```python
from build123d import *

# Parameters (mm, degrees)
SKETCH1_W               = 47
SKETCH1_H               = 26.5
SKETCH1_W_2             = 41
SKETCH1_H_2             = 20.5
BOSS_EXTRUDE1_DEPTH     = 31
CUT_EXTRUDE2_DEPTH      = 31
SKETCH4_W               = 34.29807853
SKETCH4_H               = 20
BOSS_EXTRUDE2_DEPTH     = 10
SKETCH5_W               = 5
SKETCH5_H               = 17.5
CUT_EXTRUDE3_DEPTH      = 45
CUT_EXTRUDE4_DEPTH      = 64
CUT_EXTRUDE4_DEPTH_BACK = 45
SKETCH6_R               = 4.31945574
SKETCH7_W               = 8.63891148
SKETCH7_H               = 8.75
CUT_EXTRUDE5_DEPTH      = 10
FILLET2_START           = -23.25
FILLET2_DEPTH           = 5
SKETCH8_W               = 26.5
SKETCH8_H               = 5.5
CUT_EXTRUDE6_DEPTH      = 55
BOSS_EXTRUDE3_DEPTH     = 2.4
SKETCH10_W              = 5
SKETCH10_H              = 20
CUT_EXTRUDE7_DEPTH      = 39.4
FILLET4_R               = 5


with BuildPart() as part:
    # Sketch1 → Boss-Extrude1 (new body)
    with BuildSketch(Plane(origin=(0, 0, 0), x_dir=(1, 0, 0), z_dir=(0, 1, 0))):
        Rectangle(SKETCH1_W, SKETCH1_H)
        Rectangle(SKETCH1_W_2, SKETCH1_H_2, mode=Mode.SUBTRACT)
    extrude(amount=BOSS_EXTRUDE1_DEPTH)

    # Sketch3 → Cut-Extrude2 (cut)
    with BuildSketch(Plane(origin=(0, 31, 0), x_dir=(1, 0, 0), z_dir=(0, 1, 0))):
        Polygon((-19.366144394, -10.25), (-20.5, -13.25), (0, -13.25), (0, -10.25), align=None)
        Polygon((0, -10.25), (0, -13.25), (20.5, -13.25), (19.366144394, -10.25), align=None)
    extrude(amount=-CUT_EXTRUDE2_DEPTH, mode=Mode.SUBTRACT)

    # Sketch4 → Boss-Extrude2 (add)
    with BuildSketch(Plane(origin=(0, 0, -13.25), x_dir=(-1, 0, 0), z_dir=(0, 0, -1))):
        with Locations((0, 15.5)):
            Rectangle(SKETCH4_W, SKETCH4_H)
    extrude(amount=BOSS_EXTRUDE2_DEPTH)

    # Sketch5 → Cut-Extrude3 (cut)
    with BuildSketch(Plane(origin=(17.149039265, 0, 0), x_dir=(0, 0, -1), z_dir=(1, 0, 0))):
        with Locations((15.75, 14.25)):
            Rectangle(SKETCH5_W, SKETCH5_H)
    extrude(amount=-CUT_EXTRUDE3_DEPTH, mode=Mode.SUBTRACT)

    # Sketch6 → Cut-Extrude4 (cut, two sides: drawn at the far end of the back side and taken through both)
    with BuildSketch(Plane.XY.offset(-18.25).offset(-CUT_EXTRUDE4_DEPTH_BACK)):
        with Locations(Location((0, 14.25, 0), (0, 0, 180))):
            Circle(SKETCH6_R)
    extrude(amount=CUT_EXTRUDE4_DEPTH + CUT_EXTRUDE4_DEPTH_BACK, mode=Mode.SUBTRACT)

    # Sketch7 → Cut-Extrude5 (cut)
    with BuildSketch(Plane(origin=(0, 0, -23.25), x_dir=(-1, 0, 0), z_dir=(0, 0, -1))):
        with Locations((0, 9.875)):
            Rectangle(SKETCH7_W, SKETCH7_H)
    extrude(amount=-CUT_EXTRUDE5_DEPTH, mode=Mode.SUBTRACT)

    # Fillet2: read off the stored shape, not the designer's step
    # Fillet2 outline → Fillet2 (cut)
    with BuildSketch(Plane.XY.offset(FILLET2_START)):
        with BuildLine():
            ThreePointArc((-4.31945574, 14.25), (-4.315331507, 14.438711079), (-4.302966685, 14.627061794))
            ThreePointArc((-4.302966685, 14.627061794), (-7.509401663, 8.126758445), (-14.264792768, 5.5))
            Line((-14.264792768, 5.5), (-4.31945574, 5.5))
            Line((-4.31945574, 5.5), (-4.31945574, 14.25))
        make_face()
        with BuildLine():
            ThreePointArc((14.264792768, 5.5), (7.509401663, 8.126758445), (4.302966685, 14.627061794))
            ThreePointArc((4.302966685, 14.627061794), (4.315331507, 14.438711079), (4.31945574, 14.25))
            Line((4.31945574, 14.25), (4.31945574, 5.5))
            Line((4.31945574, 5.5), (14.264792768, 5.5))
        make_face()
    extrude(amount=FILLET2_DEPTH, mode=Mode.SUBTRACT)

    # Sketch8 → Cut-Extrude6 (cut)
    with BuildSketch(Plane(origin=(23.5, 0, 0), x_dir=(0, 0, -1), z_dir=(1, 0, 0))):
        with Locations((0, 2.75)):
            Rectangle(SKETCH8_W, SKETCH8_H)
    extrude(amount=-CUT_EXTRUDE6_DEPTH, mode=Mode.SUBTRACT)

    # Sketch9 → Boss-Extrude3 (add)
    with BuildSketch(Plane.XY.offset(-18.25)):
        with BuildLine():
            Line((-17.149039265, 23), (17.149039265, 23))
            Line((17.149039265, 23), (17.149039265, 5.5))
            Line((17.149039265, 5.5), (14.264792768, 5.5))
            ThreePointArc((14.264792768, 5.5), (7.509401663, 8.126758445), (4.302966685, 14.627061794))
            ThreePointArc((4.302966685, 14.627061794), (0, 18.56945574), (-4.302966685, 14.627061794))
            ThreePointArc((-4.302966685, 14.627061794), (-7.509401663, 8.126758445), (-14.264792768, 5.5))
            Line((-14.264792768, 5.5), (-17.149039265, 5.5))
            Line((-17.149039265, 5.5), (-17.149039265, 23))
        make_face()
    extrude(amount=BOSS_EXTRUDE3_DEPTH)

    # Sketch10 → Cut-Extrude7 (cut)
    with BuildSketch(Plane(origin=(17.149039265, 0, 0), x_dir=(0, 0, -1), z_dir=(1, 0, 0))):
        with Locations((20.75, 15.5)):
            Rectangle(SKETCH10_W, SKETCH10_H)
    extrude(amount=-CUT_EXTRUDE7_DEPTH, mode=Mode.SUBTRACT)

    # Fillet4
    fillet4_edges = [part.edges().sort_by_distance(p)[0] for p in [
        (0, 25.5, -13.25),
    ]]
    fillet(fillet4_edges, radius=FILLET4_R - 0.0001)  # a hair under: the kernel refuses the full size


solid = part.part
```
Can you work these out from the model? Positions are in its coordinate system, mm. A direction names the side the tool comes from. Round coordinates to 2 decimals unless told otherwise and drop trailing zeros. Loops run counter-clockwise (first coordinate to the right, second up) from the corner with the lowest first, then second, coordinate; pieces in that order, holes last.
Item 1: Suppose I cut it at D-D, the plane y = 8. Write out the boundary of the cut face in (x, z), then the cut area to 3 significant figures.
Item 2: Please list where these lines run through material, in increasing order: L1, parallel to X at y = 16, z = -6.5; L2, parallel to Z at x = 13, y = 13.25; L3, parallel to Y at x = 0, z = -12.
Item 3: Which directions (+Z, -Z, +X, -X, +Y, -Y) give clear straight access to the entire face, cutting with the end or side of a thin tool? Please do faces 1 (the flat face through (-20.5, 18, 0)), 2 (the flat face through (17.149, 18, -16)), 3 (the cylindrical face through (7.586, 8.057, -17.067)), 4 (the flat face through (0, 23, -15)).
Item 4: Will these pins go through, and if not, where does the flat tip stop? pin 1 Ø4 at (x, y) = (8.5, 28) entering from +Z; pin 2 Ø0.8 at (x, z) = (-4, -15) entering from -Y.
Item 5: Suppose I cut it at B-B, the plane y = 17.5. Write out the boundary of the cut face in (x, z).
Item 6: Suppose I cut it at A-A, the plane z = 0.5. Write out the boundary of the cut face in (x, y).
Item 7: If we mould it in two halves opening along X, with no side actions, what happens to faces 5 (the flat face through (-17.149, 18, -16)), 6 (the flat face through (20.5, 18, 0)), 7 (the cylindrical face through (-7.43, 8.2, -17.07)), 8 (the flat face through (2, 5.5, -11))? For each: +X half, -X half, draft (parallel to the pull), parting line (faces both ways), or undercut.
Reported:
1. outline: (-23.5, -13.25) - (23.5, -13.25) - (23.5, 13.25) - (20.5, 13.25) - (19.37, 10.25) - (20.5, 10.25) - (20.5, -10.25) - (-20.5, -10.25) - (-20.5, 10.25) - (-19.37, 10.25) - (-20.5, 13.25) - (-23.5, 13.25) - close; (-17.15, -18.25) - (-7.65, -18.25) - (-7.65, -15.85) - (-17.15, -15.85) - close; (7.65, -18.25) - (17.15, -18.25) - (17.15, -15.85) - (7.65, -15.85) - close
1. area: 331 mm2
2. L1: x = -23.5 to -20.5, 20.5 to 23.5
2. L2: z = -18.25 to -15.85, -13.25 to -10.25
2. L3: y = 5.5 to 9.93, 18.57 to 31
3. face 1: +Y, -Y
3. face 2: -Z, +X, +Y, -Y
3. face 3: -Z, -Y
3. face 4: +X, -X, -Y
4. pin 1: stops at z = -10.25
4. pin 2: stops at y = 23
5. outline: (-23.5, -13.25) - (-2.85, -13.25) - (-2.85, -10.25) - (-20.5, -10.25) - (-20.5, 10.25) - (-19.37, 10.25) - (-20.5, 13.25) - (-23.5, 13.25) - close; (-17.15, -18.25) - (-2.85, -18.25) - (-2.85, -15.85) - (-17.15, -15.85) - close; (2.85, -18.25) - (17.15, -18.25) - (17.15, -15.85) - (2.85, -15.85) - close; (2.85, -13.25) - (23.5, -13.25) - (23.5, 13.25) - (20.5, 13.25) - (19.37, 10.25) - (20.5, 10.25) - (20.5, -10.25) - (2.85, -10.25) - close
6. outline: (-23.5, 5.5) - (-20.5, 5.5) - (-20.5, 31) - (-23.5, 31) - close; (20.5, 5.5) - (23.5, 5.5) - (23.5, 31) - (20.5, 31) - close
7. face 5: -X half
7. face 6: undercut
7. face 7: undercut
7. face 8: draft
